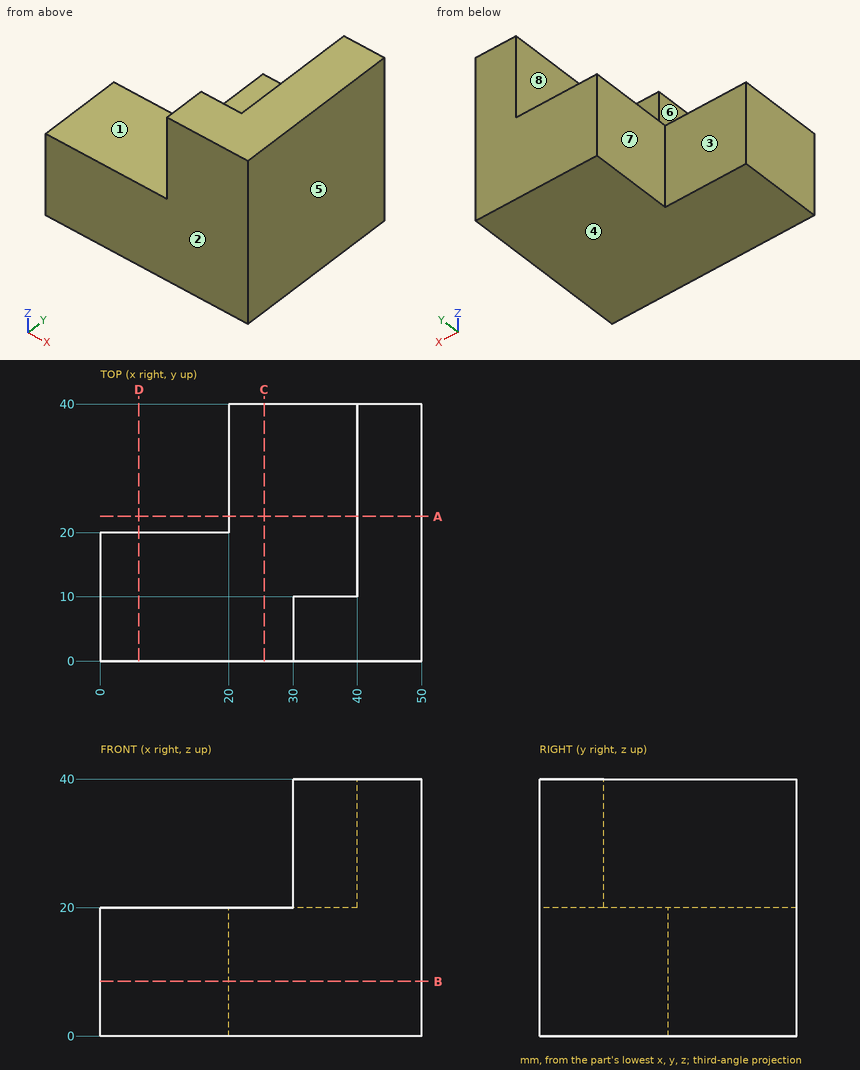
For this review, use the dimensioned drawing (mm, ordinates from the lowest corner) and the shaded views. A direction names the side the tool comes from. Round coordinates to 2 decimals unless told otherwise and drop trailing zeros. Order: outer loops, then holes, each group sorted by start corner. A loop starts at its lowest first (then second) coordinate and runs counter-clockwise, first axis right, second up. Notation, with made-up numbers: (24, 68.5) -> (51, 68.5) arc R20 cw to (51, 103.5) -> close; hole circle Ø5 at (0.5, 84). An arc over 180 degrees is marked (long way). One line per item, written item: value. Start each with the question number.
Q1. Take a section at C-C (x = 25.5). Write out the cut boundary in (y, z).
Q2. Machinability: for the marked faces 4, 5, 6, 7 and 8, which of the approach directions +Z, -Z, +X, -X, +Y, -Y give a long, thin tool a straight path to every point of the face, cutting with its end or side? Answer none if there is none.
Q3. Take a section at A-A (y = 22.5). Write out the cut boundary in (x, z).
Q4. Wall thickness on line 1 (Y direction, x = 6, z = 16); line 2 (X direction, y = 27.5, z = 22): over which ranges is each line inside the solid? List them lowest first.
Q5. Take a section at B-B (z = 8.5). Write out the cut boundary in (x, y).
Q6. Clearance check with flat-ended pins moving along their axes: pin 1 Ø8 at (x, z) = (22.5, 19.5) entering from -Y; pin 2 Ø22 at (y, z) = (18.5, 33.5) entering from -X; pin 3 Ø3 at (x, z) = (33, 25.5) entering from +Y; pin 4 Ø6 at (x, y) = (31, 33) entering from +Z. State where each tip first meets the part, or that it passes through.
Q7. Mouldability with a two-part tool opening along Y and no side actions: class the marked faces 1, 2 and 3 as released by +Y, released by -Y, zero draft, split by the parting line, or undercut.
Q8. Take a section at D-D (x = 6). Write out the cut boundary in (y, z).
Reported:
1. outline: (0, 0) -> (40, 0) -> (40, 20) -> (0, 20) -> close
2. face 4: -Z, +X, -X, +Y, -Y
2. face 5: +Z, -Z, +X, +Y, -Y
2. face 6: +Z, -X, +Y, -Y
2. face 7: +Z, -Z, -X, +Y
2. face 8: +Z, -X, +Y
3. outline: (20, 0) -> (50, 0) -> (50, 40) -> (40, 40) -> (40, 20) -> (20, 20) -> close
4. line 1: y = 0 to 20
4. line 2: x = 40 to 50
5. outline: (0, 0) -> (50, 0) -> (50, 40) -> (20, 40) -> (20, 20) -> (0, 20) -> close
6. pin 1: stops at y = 0
6. pin 2: stops at x = 30
6. pin 3: stops at y = 10
6. pin 4: stops at z = 20
7. face 1: zero draft
7. face 2: released by -Y
7. face 3: released by +Y
8. outline: (0, 0) -> (20, 0) -> (20, 20) -> (0, 20) -> close
